Source: CAD feature listing. Evaluate the final solid. Frame: model axes, mm. A direction names the side the tool comes from. Give positions to 0.01 mm unless a question says otherwise; leave off trailing zeros. Order: outer loops, then holes, each group sorted by start corner. A loop starts at its lowest first (then second) coordinate and runs counter-clockwise, first axis right, second up.
from build123d import *

# Parameters (mm, degrees)
F1_DEPTH      = 203.2
F2_W          = 25.4
F2_H          = 17.78
F3_DEPTH      = 50.8
F4_W          = 25.4
F4_H          = 17.78
F5_DEPTH      = 50.8
F11_DEPTH     = 0.0762
F31_T         = 2.54
F31_T3_DEPTH  = 30.48
F31_T5_DEPTH  = 22.86
F31_T7_DEPTH  = 157.48
F31_T9_DEPTH  = 30.48
F31_T11_DEPTH = 55.88


# Not quite as in the source:
# - a shell that OpenCascade refuses in one call is made with other operations: the cavity is built on its own and cut out
# - the program builds the solid bodies; features that only make, move or delete a surface that nothing else refers to are left out


with BuildPart() as f1:
    # F0 (on Front) → F1 (new body)
    with BuildSketch(Plane.XZ):
        Polygon((7.5239408249, -41.6093189047), (-17.8760591751, -41.6093189047), (-17.8760591751, -84.7893189047), (96.4239408249, -84.7893189047), (96.4239408249, -8.5893189047), (58.3239408249, -8.5893189047), (58.3239408249, -59.3893189047), (7.5239408249, -59.3893189047), align=None)
    extrude(amount=F1_DEPTH)

    # F2 (on face) → F3 (join)
    with BuildSketch(Plane.YZ.offset(7.5239408249)):
        with Locations((-190.5, -50.4993189047)):
            Rectangle(F2_W, F2_H)
    extrude(amount=F3_DEPTH)

    # F4 (on face) → F5 (join)
    with BuildSketch(Plane.YZ.offset(7.5239408249)):
        with Locations((-12.7, -50.4993189047)):
            Rectangle(F4_W, F4_H)
    extrude(amount=F5_DEPTH)

    # F9 (on face) → F11 (join)
    with BuildSketch(Plane(origin=(0, 0, 0), x_dir=(-1, 0, 0), z_dir=(0, 1, 0))):
        with BuildLine():
            ThreePointArc((-85.9858192503, -15.2795063332), (-92.0223010679, -14.3629027521), (-86.5299954351, -17.0300836035))
            ThreePointArc((-86.5299954351, -17.0300836035), (-86.12500001, -16.1961099143), (-85.9858192503, -15.2795063332))
        make_face()
    extrude(amount=F11_DEPTH)

    # F31: shell of thickness 2.54, made by hand


with BuildPart() as f31_core1:
    # F31_t2: copy of F1
    add(f1.part)

    # the walls: a layer under each face that stays
    f31_faces = [f31_core1.faces().sort_by_distance(p)[0] for p in [
        (77.3739408249, -101.6, -8.5893189047),
        (96.4239408249, -101.6, -46.6893189047),
        (58.3239408249, -101.6, -33.9893189047),
        (39.2739408249, 0, -46.6893189047),
        (39.2739408249, -203.2, -46.6893189047),
        (-5.1760591751, -33.8666666667, -41.6093189047),
        (32.9239408249, -25.4, -50.4993189047),
        (32.9239408249, -101.6, -59.3893189047),
        (32.9239408249, -177.8, -50.4993189047),
        (-17.8760591751, -101.6, -63.1993189047),
        (91.6173056428, 0.0381, -13.5289290629),
        (7.5239408249, -101.6, -50.4993189047),
        (89.0736505389, 0.0762, -15.2795063332),
    ]]
    thicken(f31_faces, amount=-F31_T, mode=Mode.SUBTRACT)

    # F31_s4 → F31_t3 (cut)
    with BuildSketch(Plane.XZ.offset(-2.54)):
        Polygon((58.2985408249, -41.5839189047), (60.8639408249, -41.6093189047), (60.8639408249, -44.1493189047), (58.3239408249, -44.1493189047), align=None)
    extrude(amount=F31_T3_DEPTH, mode=Mode.SUBTRACT)

    # F31_s6 → F31_t5 (cut)
    with BuildSketch(Plane.XY.offset(-61.9293189047)):
        Polygon((58.2985408249, -25.4254), (60.8639408249, -25.4), (60.8639408249, -22.86), (58.3239408249, -22.86), align=None)
        Polygon((58.2985408249, -177.7746), (60.8639408249, -177.8), (60.8639408249, -180.34), (58.3239408249, -180.34), align=None)
        Polygon((7.5493408249, -25.4254), (7.5239408249, -22.86), (4.9839408249, -22.86), (4.9839408249, -25.4), align=None)
        Polygon((7.5493408249, -177.7746), (7.5239408249, -180.34), (4.9839408249, -180.34), (4.9839408249, -177.8), align=None)
    extrude(amount=F31_T5_DEPTH, mode=Mode.SUBTRACT)

    # F31_s8 → F31_t7 (cut)
    with BuildSketch(Plane.XZ.offset(22.86)):
        Polygon((58.2985408249, -59.3639189047), (60.8639408249, -59.3893189047), (60.8639408249, -61.9293189047), (58.3239408249, -61.9293189047), align=None)
        Polygon((7.5493408249, -59.3639189047), (7.5239408249, -61.9293189047), (4.9839408249, -61.9293189047), (4.9839408249, -59.3893189047), align=None)
    extrude(amount=F31_T7_DEPTH, mode=Mode.SUBTRACT)

    # F31_s10 → F31_t9 (cut)
    with BuildSketch(Plane.XZ.offset(175.26)):
        Polygon((58.2985408249, -41.5839189047), (60.8639408249, -41.6093189047), (60.8639408249, -44.1493189047), (58.3239408249, -44.1493189047), align=None)
    extrude(amount=F31_T9_DEPTH, mode=Mode.SUBTRACT)

    # F31_s12 → F31_t11 (cut)
    with BuildSketch(Plane.YZ.offset(4.9839408249)):
        Polygon((-25.4254, -59.3639189047), (-22.86, -59.3893189047), (-22.86, -61.9293189047), (-25.4, -61.9293189047), align=None)
        Polygon((-177.7746, -59.3639189047), (-177.8, -61.9293189047), (-180.34, -61.9293189047), (-180.34, -59.3893189047), align=None)
    extrude(amount=F31_T11_DEPTH, mode=Mode.SUBTRACT)

    # F31_s13 → F31_t14 (revolve, cut)
    with BuildSketch(Plane(origin=(35.7646863661, 0, -51.9674444282), x_dir=(0, 1, 0), z_dir=(0.5669277583, 0, -0.8237675139))):
        Polygon((0.0254, 61.6003720947), (-2.54, 61.6257720947), (-2.54, 64.1657720947), (0, 64.1657720947), align=None)
    revolve(axis=Axis((89.0736505389, 0, -15.2795063332), (0, 1, 0)), mode=Mode.SUBTRACT)


with BuildPart() as f1_1:
    add(f1.part)

    # what is left inside the walls is the cavity
    f31_cavity = [f31_core1.part.solids().sort_by_distance(p)[0] for p in [
        (39.273941, -134.62, -84.763919),
    ]]
    add(f31_cavity, mode=Mode.SUBTRACT)


solid = f1_1.part
(1) Draft query along Y for faces 1 (the flat face through (-3, -103, -44.149)), 2 (the flat face through (-16, -101, -84.789)), 3 (the flat face through (51, 0, -56)). Return one class per face: +Y half, -Y half, draft (parallel to the pull), parting line (faces both ways), or undercut.
(2) Section B-B, the plane z = -72.5. Return loops of the section in (x, y), plus the area to 3 significant figures.
(3) Section A-A, the plane x = 68. Return loops of the section in (y, z).
(4) Access query for faces 4 (the flat face through (58.324, -100, -34)), 5 (the flat face through (3, -103, -41.609)), 6 (the flat face through (78, -100, -8.589)), 7 (the flat face through (93.884, -100, -48)), 8 (the flat face through (51, -203.2, -56)). Directions: +Z, -Z, +X, -X, +Y, -Y. A direction counts if a zero-diameter tool reaches every point of the face in a straight line with its end or side. Return the directions, or none.
(5) Pin query (flat end, axial travel): pin 1 Ø10 at (x, y) = (37, -147) entering from +Z; pin 2 Ø22 at (x, z) = (62, -63) entering from +Y; pin 3 Ø12 at (x, y) = (10.5, -162) entering from -Z. Return the tip coordinate at first contact, or that it passes through.
(6) Line query: line 1 along X through (y, z) = (-40.5, -60.5); line 2 along X through (y, z) = (-162, -50); line 3 along Y through (x, z) = (80.5, -33). Output: solid intervals per line, ascending.
(7) Section D-D, the plane x = -9. Return loops of the section in (y, z).
(8) Section C-C, the plane y = -57.5. Return loops of the section in (x, z).
Checks:
1. face 1: undercut
1. face 2: draft
1. face 3: +Y half
2. outline: (-17.88, -203.2) - (96.42, -203.2) - (96.42, 0) - (-17.88, 0) - close; hole (-15.34, -200.66) - (93.88, -200.66) - (93.88, -2.54) - (-15.34, -2.54) - close
2. area: 1,590 mm2
3. outline: (-203.2, -84.79) - (-200.66, -84.79) - (-200.66, -11.13) - (-2.54, -11.13) - (-2.54, -84.79) - (0, -84.79) - (0, -8.59) - (-203.2, -8.59) - close
4. face 4: +Z
4. face 5: +Z, -X, +Y, -Y
4. face 6: +Z, +X, -X, +Y, -Y
4. face 7: -Z
4. face 8: +Z, -Z, +X, -X, -Y
5. pin 1: stops at z = -59.39
5. pin 2: stops at y = 0
5. pin 3: stops at z = -61.93
6. line 1: x = -17.88 to -15.34, 4.98 to 60.86, 93.88 to 96.42
6. line 2: x = -17.88 to -15.34, 4.98 to 7.52, 58.32 to 60.86, 93.88 to 96.42
6. line 3: y = -203.2 to -200.66, -2.54 to 0
7. outline: (-203.2, -84.79) - (-200.66, -84.79) - (-200.66, -44.15) - (-2.54, -44.15) - (-2.54, -84.79) - (0, -84.79) - (0, -41.61) - (-203.2, -41.61) - close
8. outline: (-17.88, -84.79) - (-15.34, -84.79) - (-15.34, -44.15) - (4.98, -44.15) - (4.98, -61.93) - (60.86, -61.93) - (60.86, -11.13) - (93.88, -11.13) - (93.88, -84.79) - (96.42, -84.79) - (96.42, -8.59) - (58.32, -8.59) - (58.32, -59.39) - (7.52, -59.39) - (7.52, -41.61) - (-17.88, -41.61) - close
